from build123d import *

# Parameters (mm, degrees)
SKETCH_1_R          = 19.5
SKETCH_1_R_2        = 18
EXTRUDE_1_DEPTH     = 20
SKETCH_3_R          = 27.5
EXTRUDE_2_DEPTH     = 3
SKETCH_4_R          = 21.75
EXTRUDE_3_DEPTH     = 2
EXTRUDE_START       = 1
SKETCH_8_R          = 21.75
EXTRUDE_4_DEPTH     = 2
SKETCH_6_R          = 18
CUT_EXTRUDE_1_DEPTH = 35


with BuildPart() as part:
    # 草圖1 → 填料-伸長1 (new body)
    with BuildSketch(Plane(origin=(0, 0, 0), x_dir=(1, 0, 0), z_dir=(0, 1, 0))):
        Circle(SKETCH_1_R)
        Circle(SKETCH_1_R_2, mode=Mode.SUBTRACT)
    extrude(amount=EXTRUDE_1_DEPTH)

    # 草圖3 → 填料-伸長2 (add)
    with BuildSketch(Plane.XZ):
        Circle(SKETCH_3_R)
    extrude(amount=EXTRUDE_2_DEPTH)

    # 草圖4 → 填料-伸長3 (add)
    with BuildSketch(Plane(origin=(0, 8, 0), x_dir=(1, 0, 0), z_dir=(0, 1, 0))):
        Circle(SKETCH_4_R)
    extrude(amount=-EXTRUDE_3_DEPTH)

    # 草圖8 → 填料-伸長4 (add)
    with BuildSketch(Plane(origin=(0, 11.5, 0), x_dir=(1, 0, 0), z_dir=(0, 1, 0)).offset(EXTRUDE_START)):
        Circle(SKETCH_8_R)
    extrude(amount=EXTRUDE_4_DEPTH)

    # 草圖6 → 除料-伸長1 (cut)
    with BuildSketch(Plane(origin=(0, 0, 0), x_dir=(1, 0, 0), z_dir=(0, 1, 0))):
        Circle(SKETCH_6_R)
    extrude(amount=CUT_EXTRUDE_1_DEPTH, mode=Mode.SUBTRACT)


solid = part.part
Can you work these out from the model? Positions are in its coordinate system, mm. A direction names the side the tool comes from. Round coordinates to 2 decimals unless told otherwise and drop trailing zeros. Write each loop counter-clockwise with the first axis right and the second up, starting at its lowest first coordinate (ties: lowest second). Pieces come first, ordered by that corner, then holes. Notation, with made-up numbers: (-6, -23.75) -> (15, -23.75) arc R12 cw to (15, -19.75) -> close; hole circle Ø4 at (2.5, 0.5). An arc over 180 degrees is marked (long way). One line per question, with ' | ' between items. Start each with the question number.
1) On a 3-axis mill with a long thin cutter (end or side, diameter ignored), from which of +Z, -Z, +X, -X, +Y, -Y can I reach the whole of each face in a straight line? I mean faces 4 (the cylindrical face through (-2.831, 7.014, -21.565)), 5 (the flat face through (-8, 8, -18)), 6 (the flat face through (0, -3, 0)). Say none if no direction works.
2) If we mould it in two halves opening along Z, with no side actions, what happens to faces 1 (the cylindrical face through (-2.343, 9.86, -17.847)), 2 (the cylindrical face through (-5.961, -1.479, -26.846)), 3 (the flat face through (5.69, 20, 17.24))? For each: released by +Z, released by -Z, zero draft, split by the parting line, or undercut.
3) Suppose I cut it at D-D on y = 3.5. Write out the boundary of the cut face in (x, z), then the cut area to 3 significant figures.
4) I need wall thicknesses on line 1 (Y direction, x = 11.5, z = -17); line 2 (Z direction, x = 0, y = 7.5); line 3 (Z direction, x = 0, y = 9). Which ranges of each line are inside material? Lowest first, please. Write a range as [from, to].
5) Suppose I cut it at A-A on z = 0. Write out the boundary of the cut face in (x, y).
6) Suppose I cut it at B-B on x = -21. Write out the boundary of the cut face in (y, z), then the cut area to 3 significant figures.
7) Suppose I cut it at C-C on x = 0. Write out the boundary of the cut face in (y, z), then the cut area to 3 significant figures.
8) I'm going to push flat-ended pins straight in: P1, Ø1.5, axis at y = 0, z = 19.5, coming from the +X side; P2, Ø1.5, axis at x = -12, y = 2, coming from the -Z side; P3, Ø3, axis at y = 14.5, z = -5.5, coming from the +X side. Where does each tip first touch, or does it pass through?
Return value:
1) face 4: +Y | face 5: none | face 6: +Z, -Z, +X, -X, -Y
2) face 1: undercut | face 2: split by the parting line | face 3: zero draft
3) outline: circle Ø39 at (0, 0); hole circle Ø36 at (0, 0) | area: 177 mm2
4) line 1: y = [-3, 0], [6, 8], [12.5, 14.5] | line 2: z = [-21.75, -18], [18, 21.75] | line 3: z = [-19.5, -18], [18, 19.5]
5) outline: (-27.5, -3) -> (27.5, -3) -> (27.5, 0) -> (19.5, 0) -> (19.5, 6) -> (21.75, 6) -> (21.75, 8) -> (19.5, 8) -> (19.5, 12.5) -> (21.75, 12.5) -> (21.75, 14.5) -> (19.5, 14.5) -> (19.5, 20) -> (18, 20) -> (18, 0) -> (-18, 0) -> (-18, 20) -> (-19.5, 20) -> (-19.5, 14.5) -> (-21.75, 14.5) -> (-21.75, 12.5) -> (-19.5, 12.5) -> (-19.5, 8) -> (-21.75, 8) -> (-21.75, 6) -> (-19.5, 6) -> (-19.5, 0) -> (-27.5, 0) -> close
6) outline: (-3, -17.76) -> (0, -17.76) -> (0, 17.76) -> (-3, 17.76) -> close; (6, -5.66) -> (8, -5.66) -> (8, 5.66) -> (6, 5.66) -> close; (12.5, -5.66) -> (14.5, -5.66) -> (14.5, 5.66) -> (12.5, 5.66) -> close | area: 152 mm2
7) outline: (-3, -27.5) -> (0, -27.5) -> (0, -19.5) -> (6, -19.5) -> (6, -21.75) -> (8, -21.75) -> (8, -19.5) -> (12.5, -19.5) -> (12.5, -21.75) -> (14.5, -21.75) -> (14.5, -19.5) -> (20, -19.5) -> (20, -18) -> (0, -18) -> (0, 18) -> (20, 18) -> (20, 19.5) -> (14.5, 19.5) -> (14.5, 21.75) -> (12.5, 21.75) -> (12.5, 19.5) -> (8, 19.5) -> (8, 21.75) -> (6, 21.75) -> (6, 19.5) -> (0, 19.5) -> (0, 27.5) -> (-3, 27.5) -> close | area: 243 mm2
8) P1: stops at x = 20.12 | P2: stops at z = -15.93 | P3: stops at x = 21.38
